from build123d import *

# Parameters (mm, degrees)
SKETCH1_W           = 206.253
SKETCH1_H           = 253.103
BOSS_EXTRUDE1_DEPTH = 3.175
BOSS_EXTRUDE3_DEPTH = 3.175
FILLET1_R           = 0.79375


with BuildPart() as part:
    # Sketch1 → Boss-Extrude1 (new body)
    with BuildSketch(Plane.XY):
        with Locations((103.1265, 126.5515)):
            Rectangle(SKETCH1_W, SKETCH1_H)
    extrude(amount=BOSS_EXTRUDE1_DEPTH)

    # Sketch3 → Boss-Extrude3 (add)
    with BuildSketch(Plane.XY):
        with BuildLine():
            Line((90.4265, 253.103), (115.8265, 253.103))
            ThreePointArc((115.8265, 253.103), (103.1265, 265.803), (90.4265, 253.103))
        make_face()
    extrude(amount=BOSS_EXTRUDE3_DEPTH)

    # Fillet1
    fillet1_edges = [part.edges().sort_by_distance(p)[0] for p in [
        (115.8265, 253.103, 1.5875),
        (90.4265, 253.103, 1.5875),
        (0, 253.103, 1.5875),
        (206.253, 253.103, 1.5875),
        (206.253, 0, 1.5875),
        (0, 0, 1.5875),
    ]]
    fillet(fillet1_edges, radius=FILLET1_R)


solid = part.part
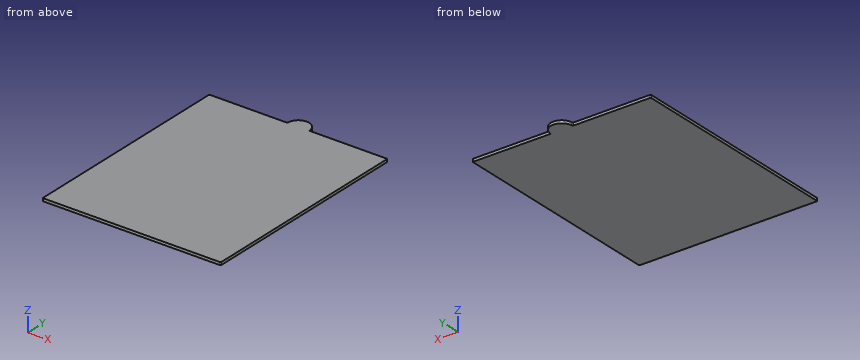
Design review of the part built by this model. Coordinates are the model's own, in mm. Round coordinates to 2 decimals unless told otherwise and drop trailing zeros. Loops run counter-clockwise (first coordinate to the right, second up) from the corner with the lowest first, then second, coordinate; pieces in that order, holes last. Notation, with made-up numbers: (77.5, 46.5) - (86.5, 46.5) arc R20 cw to (86.5, 60.5) - close; hole circle Ø2 at (5, -17). An arc over 180 degrees is marked (long way). One line per question, with ' | ' between items.
1. For L1, parallel to Y at x = 119, z = 1.6; L2, parallel to X at y = 254, z = 2.65, list the stretches that pass through material, from the lowest coordinate up. Write a range as [from, to].
Results are:
L1: y = [0, 253.1] | L2: x = [90.46, 115.79]
2. We need section A-A, the plane z = 0.6. State the section outline as (x, y) points.
Results are:
outline: (0, 0.79) arc R0.79 ccw to (0.79, 0) - (205.46, 0) arc R0.79 ccw to (206.25, 0.79) - (206.25, 252.31) arc R0.79 ccw to (205.46, 253.1) - (116.6, 253.1) arc R0.79 cw to (115.8, 253.85) arc R12.7 ccw to (90.45, 253.85) arc R0.79 cw to (89.66, 253.1) - (0.79, 253.1) arc R0.79 ccw to (0, 252.31) - close
3. We need section B-B, the plane x = 75.5. State the section outline as (y, z) points (3 decimals).
Results are:
outline: (0, 0) - (253.103, 0) - (253.103, 3.175) - (0, 3.175) - close
4. Clearance check with a flat-ended pin moving along its axis: P1, Ø1.6, axis at x = 54, z = 1, coming from the +Y side. State where the tip first meets the part, or that it passes through.
Results are:
P1: stops at y = 253.1
